CAD build for the part. Positions are in the model's coordinates, mm. A direction names the side the tool comes from. Coordinates: 2 decimals unless noted, no trailing zeros. Loops run counter-clockwise (first coordinate to the right, second up) from the corner with the lowest first, then second, coordinate; pieces in that order, holes last.
1) Saw through at B-B, the plane x = 26. Write the cut outline in (y, z).
2) Saw through at A-A, the plane y = -5.5. Write the cut outline in (x, z).
3) Which spindle directions (+Z, -Z, +X, -X, +Y, -Y) get a long thin tool onto all of the face, cutting with end or side? Do faces 1 (the flat face through (24, 7.5, 24)), 2 (the flat face through (20, 15, 15)), 3 (the flat face through (24, -7.5, 24)), 4 (the flat face through (20.28, -0.21, 7.395)), 5 (the flat face through (30, 0, 22)). Say none if no direction does.
4) Pin check, flat tips, straight feed: pin 1 Ø2 at (y, z) = (-2, 26) entering from +X; pin 2 Ø10 at (x, z) = (14, 6) entering from +Y; pin 3 Ø2 at (x, z) = (25, 22.5) entering from +Y; pin 4 Ø4 at (x, y) = (26.5, 0) entering from +Z. Stop position of each tip, or through.
5) Wall check: line 1 along Y through (x, z) = (24, 23.5); line 2 along Z through (x, y) = (33, 1.25) (3 decimals); line 3 along X through (y, z) = (-3.5, 24.25). Give the ranges that are in metal, low to high.
6) Saw through at C-C, the plane z = 6. Write the cut outline in (x, y), and give its area (3 significant figures).
7) Saw through at D-D, the plane x = 18. Write the cut outline in (y, z), and give its area (3 significant figures).
```python
from build123d import *

# Parameters (mm, degrees)
F1_DEPTH = 15
F2_DEPTH = 7.5
F3_DEPTH = 15


with BuildPart() as f1:
    # F0 (on Front) → F1 (new body, symmetric)
    with BuildSketch(Plane.XZ):
        Polygon((0, 15), (0, 0), (40, 0), align=None)
        Polygon((10, 18.75), (30, 18.75), (10, 26.25), align=None)
        Polygon((0, 15), (40, 0), (40, 15), (30, 18.75), (10, 18.75), (10, 26.25), (0, 30), align=None)
    extrude(amount=F1_DEPTH, both=True)

    # F0 (on Front) → F2 (join, symmetric)
    with BuildSketch(Plane.XZ):
        Polygon((10, 26.25), (30, 18.75), (30, 26.25), align=None)
    extrude(amount=F2_DEPTH, both=True)

    # F0 (on Front) → F3 (cut, symmetric)
    with BuildSketch(Plane.XZ):
        Polygon((0, 15), (0, 0), (40, 0), align=None)
    extrude(amount=F3_DEPTH, both=True, mode=Mode.SUBTRACT)


solid = f1.part
```
Data:
1. outline: (-15, 5.25) - (15, 5.25) - (15, 20.25) - (7.5, 20.25) - (7.5, 26.25) - (-7.5, 26.25) - (-7.5, 20.25) - (-15, 20.25) - close
2. outline: (0, 15) - (40, 0) - (40, 15) - (30, 18.75) - (30, 26.25) - (10, 26.25) - (0, 30) - close
3. face 1: +Z, +X, +Y
3. face 2: +Z, -Z, +X, -X, +Y
3. face 3: +Z, +X, -Y
3. face 4: -Z, -X, +Y, -Y
3. face 5: +Z, +X, +Y, -Y
4. pin 1: stops at x = 30
4. pin 2: stops at y = 15
4. pin 3: stops at y = 7.5
4. pin 4: stops at z = 26.25
5. line 1: y = -7.5 to 7.5
5. line 2: z = 2.625 to 17.625
5. line 3: x = 0 to 30
6. outline: (24, -15) - (40, -15) - (40, 15) - (24, 15) - close
6. area: 480 mm2
7. outline: (-15, 8.25) - (15, 8.25) - (15, 23.25) - (7.5, 23.25) - (7.5, 26.25) - (-7.5, 26.25) - (-7.5, 23.25) - (-15, 23.25) - close
7. area: 495 mm2
